```python
from build123d import *

# Parameters (mm, degrees)
EXTRUDE_1_DEPTH     = 25
SKETCH_2_R          = 1.6
CUT_EXTRUDE_1_DEPTH = 50


with BuildPart() as part:
    # ｽｹｯﾁ1 → ﾎﾞｽ - 押し出し1 (new body, symmetric)
    with BuildSketch(Plane.XY):
        Polygon((0, 0), (56.848934894, 26.509093699), (56.848934894, 46.167032185), (58.848934894, 46.167032185), (58.848934894, 25.234953177), (0.845236523, -1.812615574), align=None)
    extrude(amount=EXTRUDE_1_DEPTH, both=True)

    # ｽｹｯﾁ2 → ｶｯﾄ - 押し出し1 (cut)
    with BuildSketch(Plane(origin=(58.848934894, 0, 0), x_dir=(0, 0, -1), z_dir=(1, 0, 0))):
        with Locations((0, 36.167032185)):
            Circle(SKETCH_2_R)
    extrude(amount=-CUT_EXTRUDE_1_DEPTH, mode=Mode.SUBTRACT)


solid = part.part
```
Input: part model. Units: mm. Frame: model coordinates. A direction names the side the tool comes from. Give positions to 0.01 mm unless a question says otherwise; leave off trailing zeros. Order: outer loops, then holes, each group sorted by start corner. A loop starts at its lowest first (then second) coordinate and runs counter-clockwise, first axis right, second up.
1. Cut plane C-C (y = 27.5). Return loops of the section in (x, z).
Computed:
outline: (56.85, -25) - (58.85, -25) - (58.85, 25) - (56.85, 25) - close
2. Set-up query: faces 1 (the face through (56.849, 34, 0)), 2 (the face through (30.25, 11.9, 0.35)). Return all of +Z, -Z, +X, -X, +Y, -Y with unobstructed straight access to the full face (end or side cutting, diameter ignored); none if empty.
Computed:
face 1: +Z, -Z, -X, +Y
face 2: +Z, -Z, +X, -Y
3. Cut plane D-D (x = 25). Return loops of the section in (y, z).
Computed:
outline: (9.45, -25) - (11.66, -25) - (11.66, 25) - (9.45, 25) - close
4. Cut plane A-A (z = 0). Return loops of the section in (x, y), and give its area (3 significant figures).
Computed:
outline: (0, 0) - (0.85, -1.81) - (58.85, 25.23) - (58.85, 34.57) - (56.85, 34.57) - (56.85, 26.51) - close; (56.85, 37.77) - (58.85, 37.77) - (58.85, 46.17) - (56.85, 46.17) - close
area: 161 mm2
5. Cut plane B-B (z = -13). Return loops of the section in (x, y).
Computed:
outline: (0, 0) - (0.85, -1.81) - (58.85, 25.23) - (58.85, 46.17) - (56.85, 46.17) - (56.85, 26.51) - close
6. Line query: probe 1 along Y at (x, z) = (57.85, 0); probe 2 along X at (y, z) = (42, 3); probe 3 along Y at (x, z) = (49.5, 2). Output: solid intervals per line, ascending.
Computed:
probe 1: y = 24.77 to 34.57, 37.77 to 46.17
probe 2: x = 56.85 to 58.85
probe 3: y = 20.88 to 23.08
7. Draft query along Y for faces 3 (the face through (0.43, -0.92, 0.35)), 4 (the face through (57.86, 34.75, -0.74)), 5 (the face through (38, 17, 25)), 6 (the face through (58, 46.167, 0)). Return one class per face: released by +Y, released by -Y, zero draft, split by the parting line, or undercut.
Computed:
face 3: released by -Y
face 4: undercut
face 5: zero draft
face 6: released by +Y
8. Pin query (flat end, axial travel): pin 1 Ø3 at (x, z) = (52.5, -17.5) entering from -Y; pin 2 Ø2 at (x, z) = (28.5, 17) entering from +Y; pin 3 Ø2 at (y, z) = (4.5, -10.5) entering from -X. Return the tip coordinate at first contact, or that it passes through.
Computed:
pin 1: stops at y = 21.57
pin 2: stops at y = 13.76
pin 3: stops at x = 7.51
